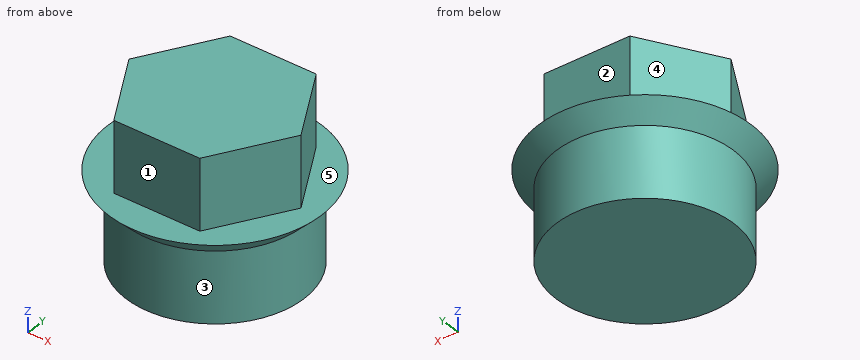
```python
from build123d import *

# Parameters (mm, degrees)
SKETCH007_R  = 5.03
PAD005_DEPTH = 5
PAD006_DEPTH = 4


with BuildPart() as part:
    # Sketch007 → Pad005 (new body)
    with BuildSketch(Plane.XY):
        Circle(SKETCH007_R)
    extrude(amount=PAD005_DEPTH)

    # Sketch008 → Pad006 (join)
    with BuildSketch(Plane.XY.offset(5)):
        Polygon((2.47, -4.278165), (4.94, 0), (2.47, 4.278165), (-2.47, 4.278165), (-4.94, 0), (-2.47, -4.278165), align=None)
    extrude(amount=PAD006_DEPTH)

    # Sketch009 → Revolution001 (revolve)
    with BuildSketch(Plane.XZ):
        Polygon((5.03, 5), (6.03, 5), (5.03, 4), align=None)
    revolve(axis=Axis((0, 0, 0), (0, 0, 1)))


solid = part.part
```
Check sheet for the modelled part. Datum: model origin and axes. Units: mm. Face numbers are marked on the shaded views. A direction names the side the tool comes from. Coordinates: 2 decimals unless noted, no trailing zeros. Write each loop counter-clockwise with the first axis right and the second up, starting at its lowest first coordinate (ties: lowest second). Pieces come first, ordered by that corner, then holes. Notation, with made-up numbers: M -7,9 L 9,9 A13 cw 9,15 Z; hole C 54.25,-13.75 d6. An arc over 180 degrees is marked long. Use one line per item in the form item = value.
Item 1: Gauge pin test, flat end, axial feed: pin 1 Ø2 at (x, z) = (0.5, 7) entering from -Y. Record the tip position at first contact, or that the pin passes through.
Answer below:
pin_1 = -4.28
Item 2: Sectioned sample at C-C, the plane z = 4.25. Record the cut outline in (x, y), and give its area (3 significant figures).
Answer below:
outline = C 0,0 d10.56
area = 87.6 mm^2
Item 3: Sectioned sample at A-A, the plane x = 0. Record the cut outline in (y, z).
Answer below:
outline = M -6.03,5 L -5.03,4 L -5.03,0 L 5.03,0 L 5.03,4 L 6.03,5 L 4.28,5 L 4.28,9 L -4.28,9 L -4.28,5 Z
Item 4: Set-up check for the marked faces 1, 2, 3, 4 and 5: record each of +Z, -Z, +X, -X, +Y, -Y from which the full face is reachable in a straight line by a thin tool's end or side.
Answer below:
face_1 = +Z, +X, -X, -Y
face_2 = +Z, +X, -X, +Y
face_3 = -Z
face_4 = +Z, -X, +Y
face_5 = +Z
Item 5: Material ranges on L1, parallel to Y at x = 0, z = 2.25; L2, parallel to Z at x = -4.75, y = 0.5; L3, parallel to X at y = 0.5, z = 7.75, recorded low to high. Write a range as from..to.
Answer below:
L1 = -5.03..5.03
L2 = 0..5
L3 = -4.65..4.65
Item 6: Sectioned sample at B-B, the plane z = 6.5. Record the cut outline in (x, y).
Answer below:
outline = M -4.94,0 L -2.47,-4.28 L 2.47,-4.28 L 4.94,0 L 2.47,4.28 L -2.47,4.28 Z
Item 7: Sectioned sample at D-D, the plane z = 2.5. Record the cut outline in (x, y), and give its area (3 significant figures).
Answer below:
outline = C 0,0 d10.06
area = 79.5 mm^2
